Answer from the drawing. Dimensions are ordinates in mm from the lowest x, y and z of the part. A direction names the side the tool comes from. Give positions to 0.01 mm unless a question says otherwise; leave off trailing zeros. Order: outer loops, then holes, each group sorted by start corner. A loop starts at its lowest first (then second) coordinate and runs counter-clockwise, first axis right, second up. Notation, with made-up numbers: (-10.5, 53.25) - (16.5, 53.25) arc R23 cw to (16.5, 88.25) - close; hole circle Ø11 at (27.25, -15). An arc over 180 degrees is marked (long way). Use a Markdown table: item, result. Add a question column.
1) Straight lines are drawn through the part: line 1 (Y direction, x = 23.5, z = 1); line 2 (Z direction, x = 13, y = 30); line 3 (Z direction, x = 16, y = 10). For each, find the intervals that lie inside material, in ascending order.
2) The mould has two halves that part along Y. Classify the marked faces 3, 4 and 5: released by +Y, released by -Y, zero draft, split by the parting line, or undercut.
3) Flat-ended cylindrical pins translate along their axes: pin 1 (6 mm diameter, centred on y = 20.5, z = 8, fed in from +X); pin 2 (6 mm diameter, centred on x = 24.49, y = 7.51, fed in from -Z); pin 3 (4.5 mm diameter, centred on x = 7.51, y = 24.49, fed in from +Z); pin 4 (1.5 mm diameter, centred on y = 9, z = 2.5, fed in from +X). Find the tip coordinate at first contact, or state that the pin passes through.
4) For the marked faces 1 and 2, determine the directions among +Z, -Z, +X, -X, +Y, -Y from which every point of the face is accessible in a straight line to the end or side of a thin tool.
5) Find section D-D, the plane z = 6.75. Determine the outline of the cut face in (x, y).
6) Find section B-B, the plane x = 16. Determine the outline of the cut face in (y, z), plus the area to 3 significant figures.
7) Find section A-A, the plane y = 16. Determine the outline of the cut face in (x, z).
8) Find section C-C, the plane z = 1. Determine the outline of the cut face in (x, y) (1 decimal).
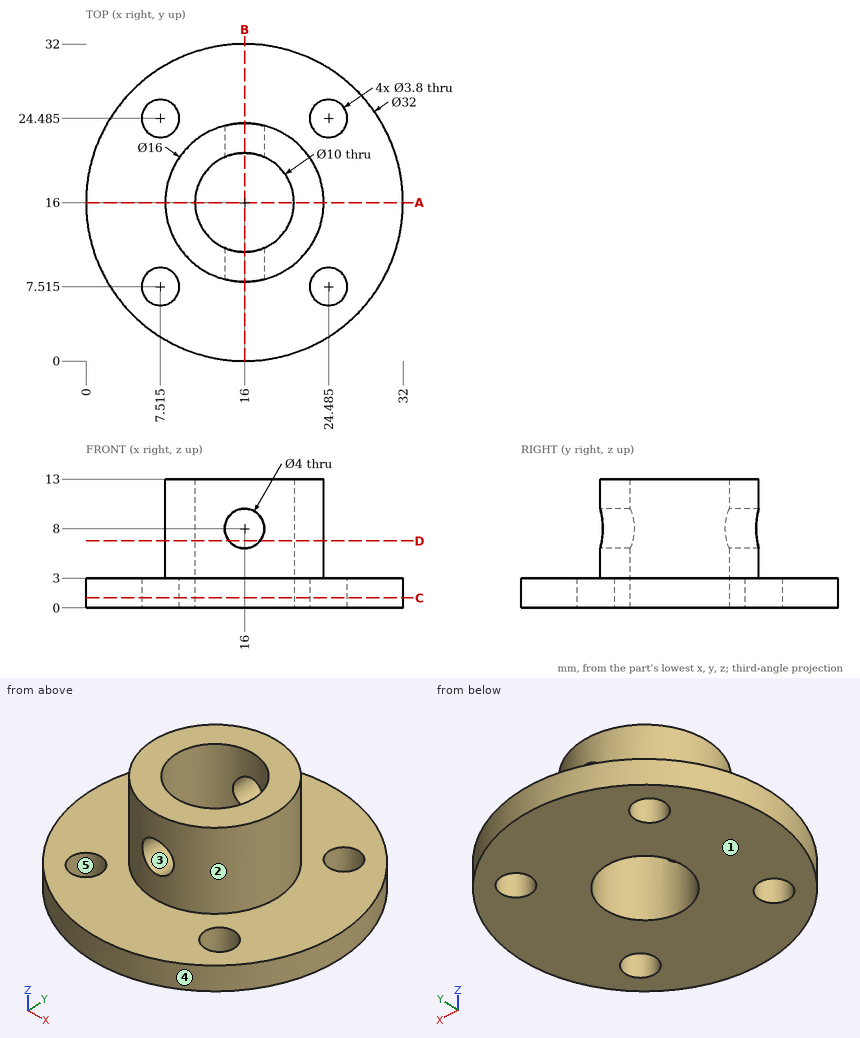
The answers:
| question | item | result |
|---|---|---|
| 1 | line 1 | 1.87 to 5.89, 9.14 to 22.86, 26.11 to 30.13 |
| 1 | line 2 | 0 to 3 |
| 1 | line 3 | 0 to 6, 10 to 13 |
| 2 | face 3 | zero draft |
| 2 | face 4 | split by the parting line |
| 2 | face 5 | undercut |
| 3 | pin 1 | x = 23.86 |
| 3 | pin 2 | z = 0 |
| 3 | pin 3 | z = 3 |
| 3 | pin 4 | x = 30.73 |
| 4 | face 1 | -Z, +X, -X, +Y, -Y |
| 4 | face 2 | +Z |
| 5 | outline | (14.44, 8.15) - (14.44, 11.25) arc R5 cw to (14.44, 20.75) - (14.44, 23.85) arc R8 ccw to start; (17.56, 8.15) arc R8 ccw to (17.56, 23.85) - (17.56, 20.75) arc R5 cw to (17.56, 11.25) - close |
| 6 | outline | (0, 0) - (11, 0) - (11, 6) - (8, 6) - (8, 3) - (0, 3) - close; (8, 10) - (11, 10) - (11, 13) - (8, 13) - close; (21, 0) - (32, 0) - (32, 3) - (24, 3) - (24, 6) - (21, 6) - close; (21, 10) - (24, 10) - (24, 13) - (21, 13) - close |
| 6 | area | 102 mm2 |
| 7 | outline | (0, 0) - (11, 0) - (11, 13) - (8, 13) - (8, 3) - (0, 3) - close; (21, 0) - (32, 0) - (32, 3) - (24, 3) - (24, 13) - (21, 13) - close |
| 8 | outline | circle Ø32 at (16, 16); hole circle Ø3.8 at (7.5, 7.5); hole circle Ø3.8 at (7.5, 24.5); hole circle Ø10 at (16, 16); hole circle Ø3.8 at (24.5, 7.5); hole circle Ø3.8 at (24.5, 24.5) |
